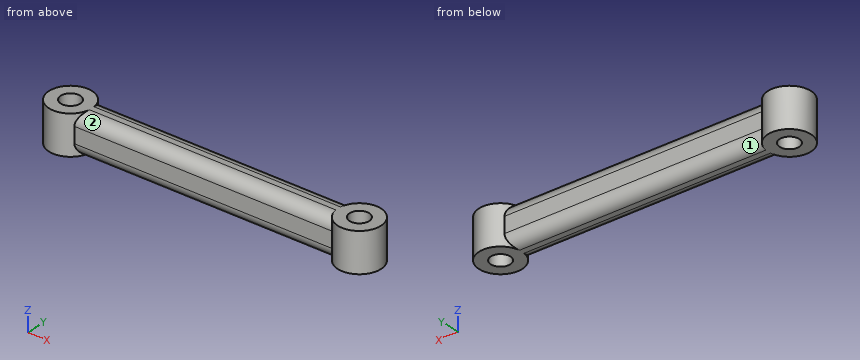
```python
from build123d import *

# Parameters (mm, degrees)
F0_R     = 1.25
F1_DEPTH = 2.5
F2_R     = 1.5


with BuildPart() as f1:
    # F0 (on Top) → F1 (new body, symmetric)
    with BuildSketch(Plane.XY):
        with BuildLine():
            ThreePointArc((2.0116846174, 1.875), (2.5587724301, 1.0075632243), (2.75, 0))
            ThreePointArc((2.75, 0), (2.5587724301, -1.0075632243), (2.0116846174, -1.875))
            Line((2.0116846174, -1.875), (34.9883153826, -1.875))
            ThreePointArc((34.9883153826, -1.875), (34.25, 0), (34.9883153826, 1.875))
            Line((34.9883153826, 1.875), (2.0116846174, 1.875))
        make_face()
        with BuildLine():
            ThreePointArc((2.0116846174, -1.875), (2.5587724301, -1.0075632243), (2.75, 0))
            ThreePointArc((2.75, 0), (2.5587724301, 1.0075632243), (2.0116846174, 1.875))
            ThreePointArc((2.0116846174, 1.875), (-2.75, 0), (2.0116846174, -1.875))
        make_face()
        Circle(F0_R, mode=Mode.SUBTRACT)
        with BuildLine():
            ThreePointArc((39.75, 0), (38.0075632243, 2.5587724301), (34.9883153826, 1.875))
            ThreePointArc((34.9883153826, 1.875), (34.25, 0), (34.9883153826, -1.875))
            ThreePointArc((34.9883153826, -1.875), (38.0075632243, -2.5587724301), (39.75, 0))
        make_face()
        with Locations((37, 0)):
            Circle(F0_R, mode=Mode.SUBTRACT)
    extrude(amount=F1_DEPTH, both=True)

    # F2
    f2_edges = [f1.edges().sort_by_distance(p)[0] for p in [
        (18.5, 1.875, 2.5),
        (18.5, -1.875, 2.5),
        (18.5, -1.875, -2.5),
        (18.5, 1.875, -2.5),
    ]]
    fillet(f2_edges, radius=F2_R)


solid = f1.part
```
Geometry check sheet. Reference: the model listing, model coordinates, mm. Face numbers are marked on the shaded views. A direction names the side the tool comes from. Round coordinates to 2 decimals unless told otherwise and drop trailing zeros. Loops run counter-clockwise (first coordinate to the right, second up) from the corner with the lowest first, then second, coordinate; pieces in that order, holes last. Notation, with made-up numbers: (51, 28.25) - (78, 28.25) arc R22 ccw to (78, 39.25) - close; hole circle Ø11 at (1.5, 4.25). An arc over 180 degrees is marked (long way). Write item = value, one per line. Start each with the question number.
1. Thickness scan on line 1 (Y direction, x = 37, z = 0.7); line 2 (X direction, y = 0.45, z = 0.2); line 3 (X direction, y = 0.55, z = -0.25). Record the ranges inside material, lowest first.
2. Set-up check for the marked faces 1 and 2: record each of +Z, -Z, +X, -X, +Y, -Y from which the full face is reachable in a straight line by a thin tool's end or side.
3. Section check C-C on z = 0.2. Enter the section's corners in (x, y) (3 decimals).
4. Section check B-B on y = 0. Enter the section's corners in (x, z).
5. Section check D-D on x = 28. Enter the section's corners in (y, z) (3 decimals), then the cut area to 3 significant figures.
6. Section check A-A on x = 37. Enter the section's corners in (y, z).
7. Depth check by flat-ended pin: pin 1 (2 mm diameter, centred on x = 13, z = 0, fed in from +Y) (3 decimals); pin 2 (1 mm diameter, centred on x = 33.5, y = 0.5, fed in from -Z); pin 3 (0.6 mm diameter, centred on x = 12, z = 0, fed in from -Y) (3 decimals). Enter the tip coordinate at first touch or a pass-through.
Working result:
q1.line_1 = -2.75 to -1.25, 1.25 to 2.75
q1.line_2 = -2.71 to -1.17, 1.17 to 35.83, 38.17 to 39.71
q1.line_3 = -2.69 to -1.12, 1.12 to 35.88, 38.12 to 39.69
q2.face_1 = -Z, +Y
q2.face_2 = +Z, -Y
q3.outline = (2.012, -1.875) - (34.988, -1.875) arc R2.75 ccw (long way) to (34.988, 1.875) - (2.012, 1.875) arc R2.75 ccw (long way) to start; hole circle Ø2.5 at (0, 0); hole circle Ø2.5 at (37, 0)
q4.outline = (-2.75, -2.5) - (-1.25, -2.5) - (-1.25, 2.5) - (-2.75, 2.5) - close; (1.25, -2.5) - (35.75, -2.5) - (35.75, 2.5) - (1.25, 2.5) - close; (38.25, -2.5) - (39.75, -2.5) - (39.75, 2.5) - (38.25, 2.5) - close
q5.outline = (-1.875, -1) arc R1.5 ccw to (-0.375, -2.5) - (0.375, -2.5) arc R1.5 ccw to (1.875, -1) - (1.875, 1) arc R1.5 ccw to (0.375, 2.5) - (-0.375, 2.5) arc R1.5 ccw to (-1.875, 1) - close
q5.area = 16.8 mm^2
q6.outline = (-2.75, -2.5) - (-1.25, -2.5) - (-1.25, 2.5) - (-2.75, 2.5) - close; (1.25, -2.5) - (2.75, -2.5) - (2.75, 2.5) - (1.25, 2.5) - close
q7.pin_1 = 1.875
q7.pin_2 = -2.5
q7.pin_3 = -1.875
